Study the drawing (mm; zero at the part's minimum x, y, z) and answer. A direction names the side the tool comes from. Give positions to 0.01 mm unless a question says otherwise; leave off trailing zeros. Order: outer loops, then holes, each group sorted by start corner. A loop starts at its lowest first (then second) coordinate and runs counter-clockwise, first axis right, second up.
Item 1: Which of the six approach directions +Z, -Z, +X, -X, +Y, -Y give full straight-line access (tool end or side, diameter ignored) to the marked faces 1 and 2?
Item 2: Given pin 1 Ø3 at (x, z) = (15.5, 88.5) entering from +Y; pin 2 Ø11.5 at (y, z) = (16.5, 147.5) entering from +X; pin 3 Ø5 at (x, y) = (9.5, 16) entering from +Z, each flat-ended and moving along its own axis, determine where each tip first touches the part or whether it passes through.
Item 3: A cutting plane is placed at B-B (x = 31). Write down the section's boundary in (y, z), plus the area to 3 significant figures.
Item 4: A cutting plane is placed at A-A (z = 115). Write down the section's boundary in (x, y), plus the area to 3 significant figures.
Item 5: Find the intervals of material crossed by line 1 along Y through (x, z) = (14.5, 49.5); line 2 along X through (y, z) = (47, 193) (1 decimal), in increasing order.
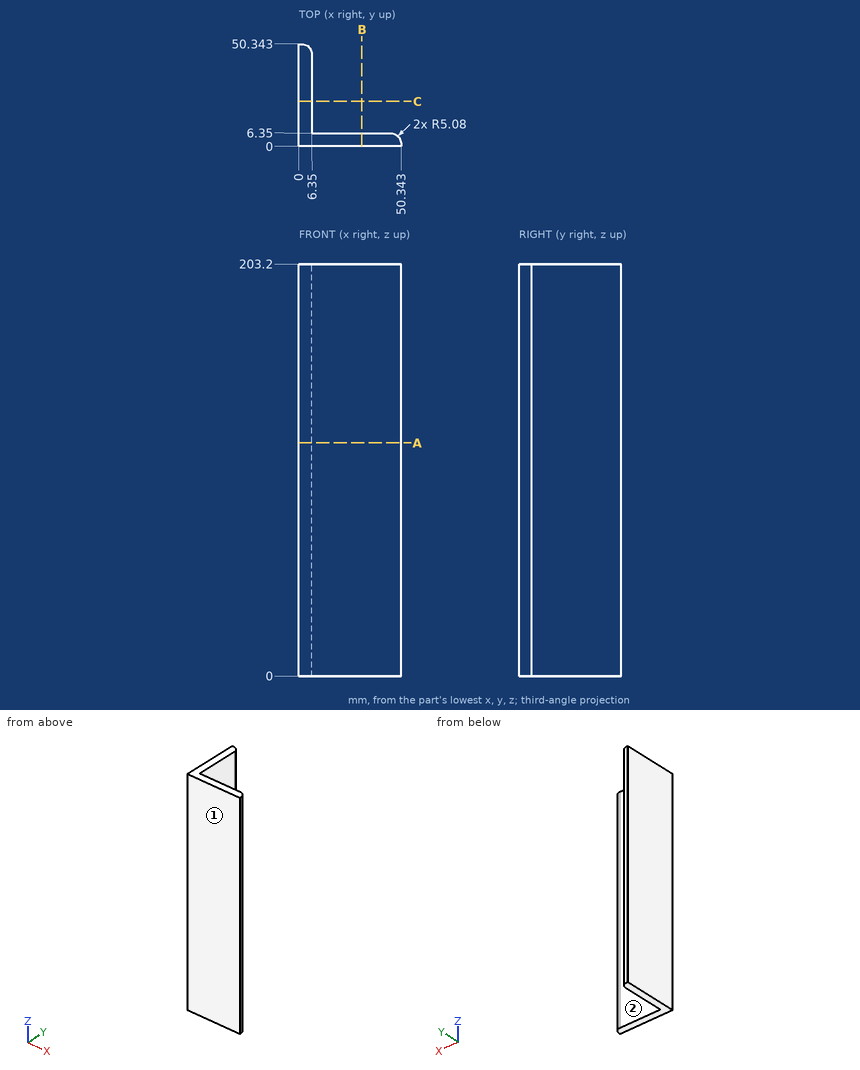
Response values:
1. face 1: +Z, -Z, +X, -X, -Y
1. face 2: +Z, -Z, +X, +Y
2. pin 1: stops at y = 6.35
2. pin 2: stops at x = 6.35
2. pin 3: passes through
3. outline: (0, 0) - (6.35, 0) - (6.35, 203.2) - (0, 203.2) - close
3. area: 1,290 mm2
4. outline: (0, 0) - (50.34, 0) - (50.34, 1.27) arc R5.08 ccw to (45.26, 6.35) - (6.35, 6.35) - (6.35, 45.26) arc R5.08 ccw to (1.27, 50.34) - (0, 50.34) - close
4. area: 588 mm2
5. line 1: y = 0 to 6.35
5. line 2: x = 0 to 6
